from build123d import *

# Parameters (mm, degrees)
F1_DEPTH = 12.9
F2_R     = 17.5
F3_DEPTH = 10
F4_R     = 13.9355
F5_DEPTH = 10


with BuildPart() as f1:
    # F0 (on Front) → F1 (new body)
    with BuildSketch(Plane.XZ):
        Polygon((-13.491611, -11.113448), (0, -11.113448), (9.827, -11.113448), (9.827, -9.355818), (10.943413, -9.355818), (10.943413, -7.737426), (8.289084, -6.434524), (8.289084, -5.843352), (9.827, -5.457411), (9.827, -3.530073), (7.544932, -1.963569), (5.381204, -0.478298), (5.261175, 0), (5.69396, 1.623498), (7.544932, 2.088001), (9.09538, 6.213676), (9.09538, 10.447838), (5.261175, 14.860648), (-0.365813, 19.485754), (0, 20.018667), (3.075247, 20.018667), (5.29399, 18.955297), (5.698295, 17.344206), (7.544932, 17.344206), (8.289084, 16.83339), (9.09538, 18.007995), (9.09538, 18.955297), (9.827, 18.453084), (10.943413, 18.733248), (11.211763, 19.124179), (10.943413, 20.193515), (10.943413, 21.15518), (10.943413, 21.767149), (10.943413, 22.991084), (9.282355, 25.65752), (4.036912, 28.848497), (2.987823, 30.684402), (-1.033684, 32.476597), (-1.033684, 33.919092), (-3.738808, 34.642849), (-5.1175, 34.296865), (-5.254929, 34.844498), (-6.453976, 35.667572), (-8.202457, 35.667572), (-9.967883, 36.078834), (-9.557529, 34.443635), (-14.647621, 26.313199), (-14.647621, 24.636446), (-14.234716, 22.991084), (-11.349722, 11.494819), (-11.349722, 8.609826), (-14.5407, 5.943392), (-14.5407, 4.544607), (-9.38268, 1.003933), (-9.38268, -0.307428), (-13.491611, -3.14871), (-13.491611, -4.634919), (-12.704795, -5.552872), (-12.704795, -6.470824), (-14.934109, -7.388777), (-14.934109, -9.355818), (-13.491611, -9.355818), align=None)
    extrude(amount=F1_DEPTH)

    # F2 (on face) → F3 (join)
    with BuildSketch(Plane(origin=(0, 0, -11.113448), x_dir=(1, 0, 0), z_dir=(0, 0, -1))):
        with Locations((-1.832305, 6.564944)):
            Circle(F2_R)
    extrude(amount=F3_DEPTH)

    # F4 (on face) → F5 (join)
    with BuildSketch(Plane(origin=(0, 0, -21.113448), x_dir=(1, 0, 0), z_dir=(0, 0, -1))):
        with Locations((-1.832305, 6.564944)):
            Circle(F4_R)
    extrude(amount=F5_DEPTH)


solid = f1.part
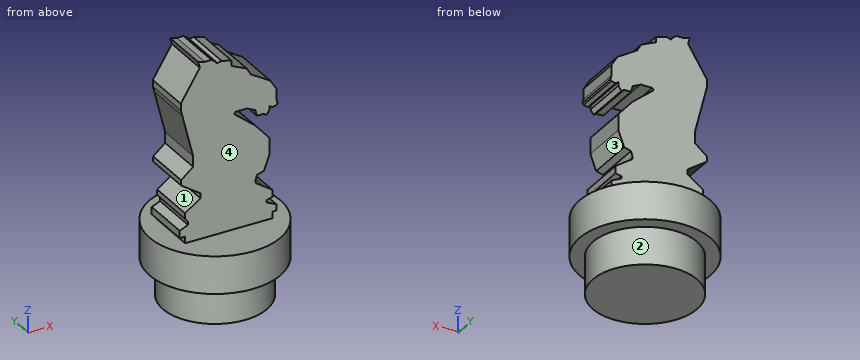
Model file for the job. Use its own axes, mm. Face numbers are marked on the shaded views. A direction names the side the tool comes from. Coordinates: 2 decimals unless noted, no trailing zeros. Order: outer loops, then holes, each group sorted by start corner. A loop starts at its lowest first (then second) coordinate and runs counter-clockwise, first axis right, second up. Notation, with made-up numbers: M 27,47 L 72,47 A21 cw 72,62 Z; hole C -8.5,68 d3. An arc over 180 degrees is marked long. Return JSON: item names as keys, results as strings.
1. Saw through at B-B (y = 5.5). Give the cut face in (x, z), and give its area (3 significant figures).
Ans:
{"outline": "M -14.51,-21.11 L -8.81,-21.11 L -8.81,-31.11 L 5.14,-31.11 L 5.14,-21.11 L 10.84,-21.11 L 10.84,-11.11 L -14.51,-11.11 Z", "area": "393 mm^2"}
2. Saw through at C-C (z = -16). Give the cut face in (x, y), and give its area (3 significant figures).
Ans:
{"outline": "C -1.83,-6.56 d35", "area": "962 mm^2"}
3. Flat gauge pins, fed straight in: pin 1 (8 mm diameter, centred on y = 5.5, z = 17, fed in from +X); pin 2 (2 mm diameter, centred on y = -9.5, z = -8.5, fed in from -X); pin 3 (0.5 mm diameter, centred on y = -8.5, z = -8, fed in from +X); pin 4 (13 mm diameter, centred on x = -2, z = 6.5, fed in from -Y). Where does each tip first touch, or does it go through?
Ans:
{"pin 1": "through", "pin 2": "x = -14.93", "pin 3": "x = 10.94", "pin 4": "y = -12.9"}
4. Saw through at A-A (x = -2.5). Give the cut face in (y, z), and give its area (3 significant figures).
Ans:
{"outline": "M -24.05,-21.11 L -20.48,-21.11 L -20.48,-31.11 L 7.35,-31.11 L 7.35,-21.11 L 10.92,-21.11 L 10.92,-11.11 L 0,-11.11 L 0,34.31 L -12.9,34.31 L -12.9,-11.11 L -24.05,-11.11 Z", "area": "1,210 mm^2"}
5. Drill centre lines: probe 1 along Z at (x, y) = (7.5, -4); probe 2 along X at (y, z) = (-6.5, -28); probe 3 along Z at (x, y) = (3, -5). Where is each one in solid material? Low to high.
Ans:
{"probe 1": "-31.11 to -1.93, 2.08 to 12.28, 17.34 to 26.74", "probe 2": "-15.77 to 12.1", "probe 3": "-31.11 to 16.72, 20.02 to 30.66"}
6. Tool access for the marked faces 1, 2, 3 and 4: list every direction of +Z, -Z, +X, -X, +Y, -Y with a clear straight run to the whole face (end or side of a thin tool).
Ans:
{"face 1": "-X, +Y, -Y", "face 2": "-Z", "face 3": "+X, +Y, -Y", "face 4": "+Z, +X, -X, -Y"}
7. Saw through at D-D (y = -16). Give the cut face in (x, z), and give its area (3 significant figures).
Ans:
{"outline": "M -16.57,-21.11 L -12.09,-21.11 L -12.09,-31.11 L 8.42,-31.11 L 8.42,-21.11 L 12.91,-21.11 L 12.91,-11.11 L -16.57,-11.11 Z", "area": "500 mm^2"}
